Work out the finished part from the listing and answer in its coordinate system (mm). Coordinates: 2 decimals unless noted, no trailing zeros. Loops run counter-clockwise (first coordinate to the right, second up) from the corner with the lowest first, then second, coordinate; pieces in that order, holes last. Notation, with made-up numbers: (16.25, 83) -> (28.25, 83) arc R17 ccw to (28.25, 87) -> close; hole circle Ø7 at (82, -34.75). An arc over 180 degrees is marked (long way). Answer as CSV lines item,"result".
```python
from build123d import *


with BuildPart() as part:
    # Sketch1 → Revolve1 (revolve)
    with BuildSketch(Plane.XY):
        Polygon((0, 0), (0, 3.81), (50.8, 3.81), (50.8, 0), (37.892541774, 0), (12.907458226, 0), align=None)
    revolve(axis=Axis((0, 3.81, 0), (1, 0, 0)))

    # Sketch6 → M3 Clearance Hole1 (revolve, cut)
    with BuildSketch(Plane.ZX.offset(3.81)):
        Polygon((0, 0), (0, 7.371463052), (1.7, 6.35), (1.7, 0), align=None)
    m3_clearance_hole1 = revolve(axis=Axis((-6.35, 3.81, 0), (1, 0, 0)), mode=Mode.SUBTRACT)

    # Mirror1: M3 Clearance Hole1 across plane
    add(m3_clearance_hole1.mirror(Plane.ZY.offset(-25.4)), mode=Mode.SUBTRACT)


solid = part.part
```
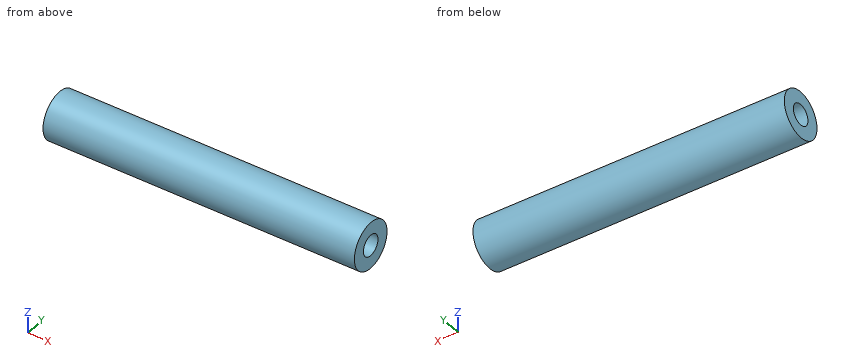
(1) Consider line 1 along Y through (x, z) = (46, 0); line 2 along Z through (x, y) = (3.5, 3.81); line 3 along Y through (x, z) = (8, -0.25). Determine where each line is inside the solid, lowest interval first.
Computed values:
line 1,"0 to 2.11, 5.51 to 7.62"
line 2,"-3.81 to -1.7, 1.7 to 3.81"
line 3,"0.01 to 7.61"
(2) A cutting plane is placed at B-B, the plane y = 6.75. Write down the section's boundary in (x, z), and give its area (3 significant figures).
Computed values:
outline,"(0, -2.42) -> (50.8, -2.42) -> (50.8, 2.42) -> (0, 2.42) -> close"
area,"246 mm2"
(3) Flat-ended cylindrical pins translate along their axes: pin 1 Ø2 at (x, z) = (19, 2.5) entering from -Y; pin 2 Ø4 at (x, y) = (20.5, 6) entering from +Z. Find the tip coordinate at first contact, or state that the pin passes through.
Computed values:
pin 1,"y = 0.31"
pin 2,"z = 3.81"
(4) A cutting plane is placed at A-A, the plane x = 20.5. Write down the section's boundary in (y, z).
Computed values:
outline,"circle Ø7.62 at (3.81, 0)"
